Could you check a few things on this model? Use its own coordinates, in mm. Face numbers are marked on the shaded views. A direction names the side the tool comes from. Coordinates: 2 decimals unless noted, no trailing zeros. Loops run counter-clockwise (first coordinate to the right, second up) from the corner with the lowest first, then second, coordinate; pieces in that order, holes last. Notation, with made-up numbers: (58.5, -20) -> (100.5, -20) arc R12 ccw to (100.5, -11) -> close; hole circle Ø4 at (62.25, 17.25). An arc over 180 degrees is marked (long way). One line per question, with ' | ' between items. Start each with the question number.
(1) If we mould it in two halves opening along Y, with no side actions, what happens to the marked faces 1, 2 and 3? For each: pulls with the +Y half, pulls with the -Y half, needs draft (parallel to the pull), parting line crosses it, or undercut.
(2) Suppose I cut it at B-B (y = -2.5). Please give me the cut outline in (x, z), plus the area to 3 significant figures.
(3) I'm going to push flat-ended pins straight in: pin 1 Ø5 at (y, z) = (-4, 12.5) entering from +X; pin 2 Ø3 at (y, z) = (-7.5, 6) entering from +X; pin 3 Ø4 at (x, y) = (9.5, -8) entering from +Z. Where does each tip first touch, or does it pass through?
(4) If I drill on line 1 along Y through (x, z) = (5, 6.75); line 2 along Z through (x, y) = (4.25, -2.5); line 3 along Z through (x, y) = (10.5, -11), over which ranges is the centre line in solid material (lowest first)?
(5) Which directions (+Z, -Z, +X, -X, +Y, -Y) give clear straight access to the entire face, cutting with the end or side of a thin tool? Please do the marked faces 4, 5 and 6.
```python
from build123d import *

# Parameters (mm, degrees)
F0_W     = 20
F0_H     = 2
F0_H_2   = 8.5
F1_DEPTH = 3
F2_DEPTH = 16
F3_R     = 0.99999


# Not quite as in the source:
# - a fillet or chamfer is up to 0.001 mm smaller than in the source, because OpenCascade refuses the exact size


with BuildPart() as f1:
    # F0 (on Top) → F1 (new body)
    with BuildSketch(Plane.XY):
        with Locations((10, -1)):
            Rectangle(F0_W, F0_H)
        with Locations((10, -6.25)):
            Rectangle(F0_W, F0_H_2)
        with Locations((10, -11.5)):
            Rectangle(F0_W, F0_H)
    extrude(amount=F1_DEPTH)

    # F0 (on Top) → F2 (join)
    with BuildSketch(Plane.XY):
        with Locations((10, -1)):
            Rectangle(F0_W, F0_H)
        with Locations((10, -11.5)):
            Rectangle(F0_W, F0_H)
    extrude(amount=F2_DEPTH)

    # F3 (radius 1 in the source; OpenCascade refuses exactly that, so slightly less here)
    f3_edges = [f1.edges().sort_by_distance(p)[0] for p in [
        (10, 0, 16),
        (0, -1, 16),
        (10, -2, 16),
        (20, -1, 16),
        (10, -10.5, 16),
        (0, -11.5, 16),
        (10, -12.5, 16),
        (20, -11.5, 16),
        (0, -6.25, 0),
        (0, 0, 8),
        (0, -2, 9.5),
        (0, -6.25, 3),
        (0, -10.5, 9.5),
        (0, -12.5, 8),
        (20, -6.25, 0),
        (20, -12.5, 8),
        (20, -10.5, 9.5),
        (20, -6.25, 3),
        (20, -2, 9.5),
        (20, 0, 8),
        (10, 0, 0),
        (10, -12.5, 0),
    ]]
    fillet(f3_edges, radius=F3_R)


solid = f1.part
```
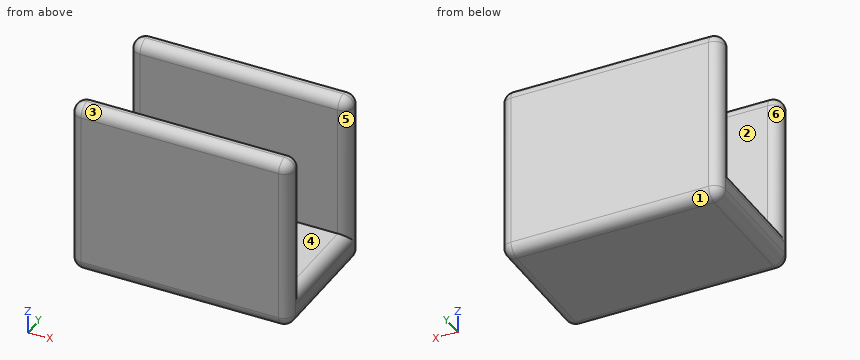
Checks:
1) face 1: pulls with the +Y half | face 2: undercut | face 3: pulls with the -Y half
2) outline: (0, 1) arc R1 ccw to (1, 0) -> (19, 0) arc R1 ccw to (20, 1) -> (20, 2) arc R1 ccw to (19, 3) -> (1, 3) arc R1 ccw to (0, 2) -> close | area: 59.1 mm^2
3) pin 1: stops at x = 19.87 | pin 2: passes through | pin 3: stops at z = 3
4) line 1: y = -12.5 to -10.5, -2 to 0 | line 2: z = 0 to 3 | line 3: z = 0 to 15.87
5) face 4: +Z, +X, -X | face 5: +Z, +X | face 6: +Z, -X
